Source: CAD feature listing. Evaluate the final solid. Frame: model axes, mm. A direction names the side the tool comes from. Coordinates: 2 decimals unless noted, no trailing zeros. Order: outer loops, then holes, each group sorted by start corner. A loop starts at its lowest first (then second) coordinate and runs counter-clockwise, first axis right, second up. Notation, with made-up numbers: (-20.75, 2.5) -> (10.25, 2.5) arc R11 ccw to (10.25, 15.5) -> close; hole circle Ø3 at (36, 53). An arc over 180 degrees is marked (long way). Write item = value, one per line. Start each with the question number.
Item 1: Section query A-A (y = 0). Output: boundary loops of the cut face in (x, z).
Item 2: Ray query, line 1 along Z through (x, y) = (3.5, -0.5); line 2 along Y through (x, z) = (33.5, 43); line 3 along Y through (x, z) = (-22.5, 12.5). Return the intervals inside material, ascending. Write a range as [from, to].
Item 3: Contact query for flat-ended pins moving along their axis: pin 1 (3 mm diameter, centred on x = 48.5, y = -19.5, fed in from -Z); pin 2 (6 mm diameter, centred on x = 50, z = 13, fed in from +Y); pin 3 (4 mm diameter, centred on y = -51.5, z = 37, fed in from +X). Output: stop coordinate, or through.
Item 4: Section query C-C (z = 21.5). Output: boundary loops of the cut face in (x, y).
Item 5: Mould query, pull axis X, two halves, no side actions, for faces 3 (the flat face through (29.2, -32.5, 0)), 4 (the flat face through (49, -17, 47.498)). Classes: released by +X, released by -X, zero draft, split by the parting line, or undercut.
Item 6: Set-up query: faces 1 (the flat face through (-1, 1, 61.468)), 2 (the flat face through (56.701, -18, 25)). Return all of +Z, -Z, +X, -X, +Y, -Y with unobstructed straight access to the full face (end or side cutting, diameter ignored); none if empty.
```python
from build123d import *

# Parameters (mm, degrees)
F0_R     = 74.761682
F1_DEPTH = 61.468
F2_R     = 43.4135
F3_DEPTH = 51.054
F4_R     = 30.660512
F5_W     = 36.541538
F5_H     = 9.436814
F6_DEPTH = 47.498


with BuildPart() as f1:
    # F0 (on Top) → F1 (new body)
    with BuildSketch(Plane.XY):
        Circle(F0_R)
    extrude(amount=F1_DEPTH)

    # F2 (on Top) → F3 (cut)
    with BuildSketch(Plane.XY):
        Circle(F2_R)
    extrude(amount=F3_DEPTH, mode=Mode.SUBTRACT)

    # F4
    f4_edges = [f1.edges().sort_by_distance(p)[0] for p in [
        (-74.761682, 0, 0),
        (-74.761682, 0, 61.468),
    ]]
    fillet(f4_edges, radius=F4_R)

    # F5 (on Top) → F6 (cut)
    with BuildSketch(Plane.XY):
        with Locations((38.430351, -17.557447)):
            Rectangle(F5_W, F5_H)
    extrude(amount=F6_DEPTH, mode=Mode.SUBTRACT)


solid = f1.part
```
Computed:
q1.outline = (-74.76, 30.66) arc R30.66 ccw to (-44.1, 0) -> (-43.41, 0) -> (-43.41, 51.05) -> (43.41, 51.05) -> (43.41, 0) -> (44.1, 0) arc R30.66 ccw to (74.76, 30.66) -> (74.76, 30.81) arc R30.66 ccw to (44.1, 61.47) -> (-44.1, 61.47) arc R30.66 ccw to (-74.76, 30.81) -> close
q2.line_1 = [51.05, 61.47]
q2.line_2 = [-64, -27.61], [27.61, 64]
q2.line_3 = [-65.02, -37.13], [37.13, 65.02]
q3.pin_1 = 47.5
q3.pin_2 = 51.8
q3.pin_3 = 55.26
q4.outline = circle Ø146.72 at (0, 0); hole (37.26, -22.28) -> (56.7, -22.28) -> (56.7, -12.84) -> (41.47, -12.84) arc R43.41 ccw (long way) to start
q5.face_3 = zero draft
q5.face_4 = undercut
q6.face_1 = +Z, +X, -X, +Y, -Y
q6.face_2 = -Z
